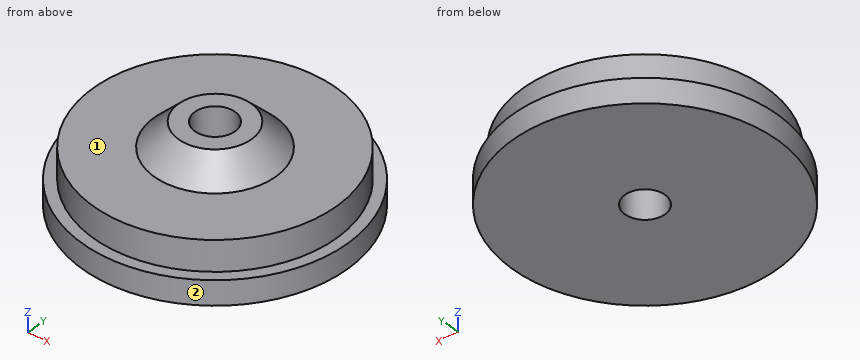
from build123d import *

# Parameters (mm, degrees)
SKETCH1_R           = 10.9
BOSS_EXTRUDE1_DEPTH = 2
SKETCH2_R           = 10
BOSS_EXTRUDE2_DEPTH = 2.5
SKETCH4_R           = 3
BOSS_EXTRUDE3_DEPTH = 2
SKETCH3_R           = 1.65
CUT_EXTRUDE1_DEPTH  = 17.729315587
CHAMFER1_SIZE       = 2


with BuildPart() as part:
    # Sketch1 → Boss-Extrude1 (new body)
    with BuildSketch(Plane.XY):
        Circle(SKETCH1_R)
    extrude(amount=BOSS_EXTRUDE1_DEPTH)

    # Sketch2 → Boss-Extrude2 (add)
    with BuildSketch(Plane.XY.offset(2)):
        Circle(SKETCH2_R)
    extrude(amount=BOSS_EXTRUDE2_DEPTH)

    # Sketch4 → Boss-Extrude3 (add)
    with BuildSketch(Plane.XY.offset(4.5)):
        Circle(SKETCH4_R)
    extrude(amount=BOSS_EXTRUDE3_DEPTH)

    # Sketch3 → Cut-Extrude1 (cut, through all)
    with BuildSketch(Plane(origin=(0, 0, 0), x_dir=(-1, 0, 0), z_dir=(0, 0, -1))):
        Circle(SKETCH3_R)
    extrude(amount=-CUT_EXTRUDE1_DEPTH, mode=Mode.SUBTRACT)

    # Chamfer1
    chamfer1_edges = [part.edges().sort_by_distance(p)[0] for p in [
        (-3, 0, 4.5),
    ]]
    chamfer(chamfer1_edges, length=CHAMFER1_SIZE - 0.0001)  # a hair under: the kernel refuses the full size


solid = part.part
Input: part model. Units: mm. Frame: model coordinates. Face numbers are marked on the shaded views. A direction names the side the tool comes from. Give positions to 0.01 mm unless a question says otherwise; leave off trailing zeros. Order: outer loops, then holes, each group sorted by start corner. A loop starts at its lowest first (then second) coordinate and runs counter-clockwise, first axis right, second up. Notation, with made-up numbers: (85, 65.25) - (131, 65.25) arc R17 ccw to (131, 81.25) - close; hole circle Ø6 at (23.5, 1.25). An arc over 180 degrees is marked (long way). Write each question's results on one line, items separated by ' | '.
Item 1: Contact query for flat-ended pins moving along their axis: pin 1 Ø6 at (x, y) = (-5, -7) entering from +Z; pin 2 Ø2 at (y, z) = (2, 0.5) entering from -X; pin 3 Ø3 at (x, z) = (5.5, 5) entering from +Y. Output: stop coordinate, or through.
A:
pin 1: stops at z = 4.5 | pin 2: stops at x = -10.85 | pin 3: stops at y = 9.13
Item 2: Access query for the marked faces 1 and 2. Directions: +Z, -Z, +X, -X, +Y, -Y. A direction counts if a zero-diameter tool reaches every point of the face in a straight line with its end or side. Return the directions, or none.
A:
face 1: +Z | face 2: +Z, -Z
Item 3: Section D-D (y = -9.5). Return loops of the section in (x, z).
A:
outline: (-5.34, 0) - (5.34, 0) - (5.34, 2) - (3.12, 2) - (3.12, 4.5) - (-3.12, 4.5) - (-3.12, 2) - (-5.34, 2) - close
Item 4: Section C-C (x = 6). Return loops of the section in (y, z).
A:
outline: (-9.1, 0) - (9.1, 0) - (9.1, 2) - (8, 2) - (8, 4.5) - (-8, 4.5) - (-8, 2) - (-9.1, 2) - close
Item 5: Material intervals for line 1 along Y through (x, z) = (0, 1.75); line 2 along Y through (x, z) = (0, 2.75); line 3 along Z through (x, y) = (7, -2.75), sorted ascending.
A:
line 1: y = -10.9 to -1.65, 1.65 to 10.9 | line 2: y = -10 to -1.65, 1.65 to 10 | line 3: z = 0 to 4.5
